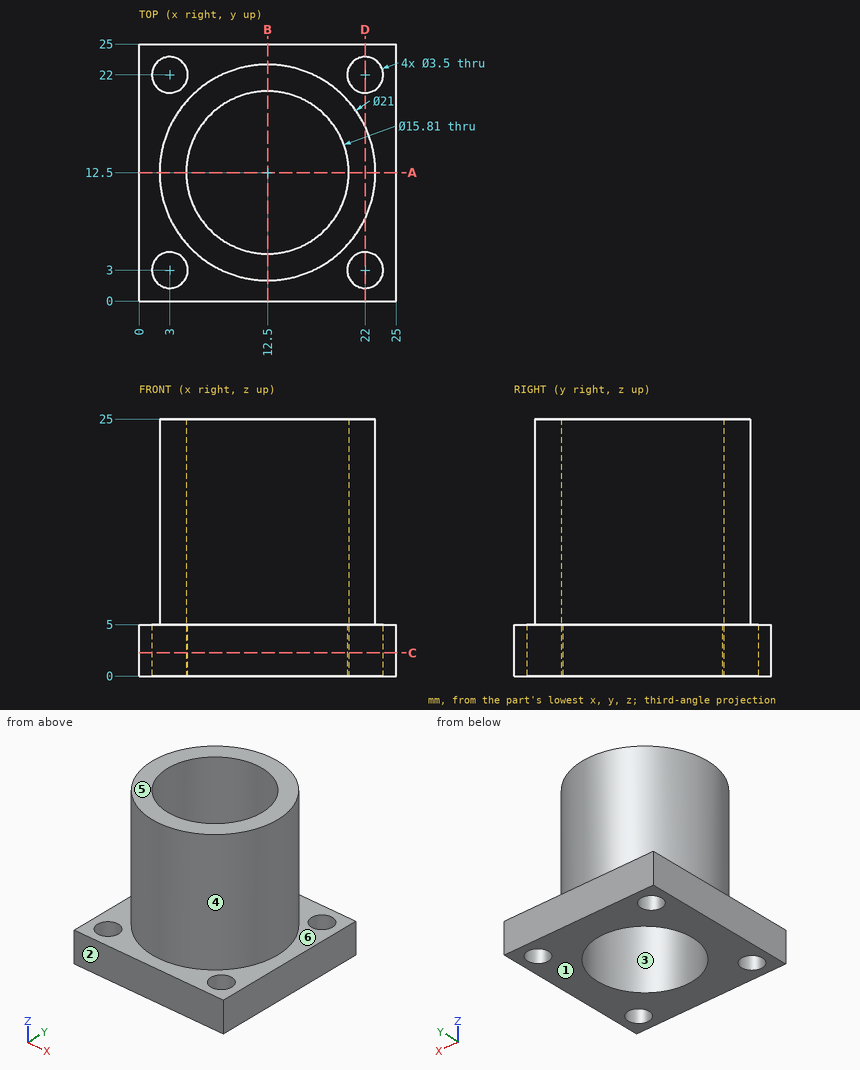
Verification items for this drawing (mm, ordinates from the low corner). A direction names the side the tool comes from. Give positions to 0.01 mm unless a question says otherwise; leave off trailing zeros. Order: outer loops, then holes, each group sorted by start corner. A loop starts at its lowest first (then second) coordinate and runs counter-clockwise, first axis right, second up. Notation, with made-up numbers: M 26,43.5 L 70,43.5 A21 ccw 70,47.5 Z; hole C -31,-24.5 d4. An arc over 180 degrees is marked long. Use a Markdown table: item, result.
Item 1: Tool access check on the marked faces 5 and 6. Record the directions out of +Z, -Z, +X, -X, +Y, -Y that give a thin tool (end or side, any length) a straight path to the whole face; none if there is none.
Answers follow:
| item | result |
|---|---|
| face 5 | +Z, +X, -X, +Y, -Y |
| face 6 | +Z |
Item 2: Section check D-D (x = 22). Record the cut outline in (y, z), and give its area (3 significant figures).
Answers follow:
| item | result |
|---|---|
| outline | M 0,0 L 1.25,0 L 1.25,5 L 0,5 Z; M 4.75,0 L 20.25,0 L 20.25,5 L 16.97,5 L 16.97,25 L 8.03,25 L 8.03,5 L 4.75,5 Z; M 23.75,0 L 25,0 L 25,5 L 23.75,5 Z |
| area | 269 mm2 |
Item 3: Section check C-C (z = 2.25). Record the cut outline in (x, y) (3 decimals).
Answers follow:
| item | result |
|---|---|
| outline | M 0,0 L 25,0 L 25,25 L 0,25 Z; hole C 3,3 d3.5; hole C 3,22 d3.5; hole C 12.5,12.5 d15.81; hole C 22,3 d3.5; hole C 22,22 d3.5 |
Item 4: Section check A-A (y = 12.5). Record the cut outline in (x, z) (3 decimals).
Answers follow:
| item | result |
|---|---|
| outline | M 0,0 L 4.595,0 L 4.595,25 L 2,25 L 2,5 L 0,5 Z; M 20.405,0 L 25,0 L 25,5 L 23,5 L 23,25 L 20.405,25 Z |
Item 5: Depth check by flat-ended pin: P1, Ø5, axis at y = 13, z = 17, coming from the +X side; P2, Ø1.5, axis at x = 22, y = 5.5, coming from the +Z side; P3, Ø2, axis at x = 11, z = 18, coming from the -Y side; P4, Ø12.5, axis at x = 12.5, y = 12.5, coming from the -Z side. Enter the tip coordinate at first touch or a pass-through.
Answers follow:
| item | result |
|---|---|
| P1 | stops at x = 23 |
| P2 | stops at z = 5 |
| P3 | stops at y = 2.01 |
| P4 | passes through |
Item 6: Material ranges on line 1 along Y through (x, z) = (3, 2); line 2 along Y through (x, z) = (1.5, 2.5); line 3 along Y through (x, z) = (12.5, 13) (3 decimals), recorded low to high.
Answers follow:
| item | result |
|---|---|
| line 1 | y = 0 to 1.25, 4.75 to 20.25, 23.75 to 25 |
| line 2 | y = 0 to 2.1, 3.9 to 21.1, 22.9 to 25 |
| line 3 | y = 2 to 4.595, 20.405 to 23 |
Item 7: Draft check along Y on the marked faces 1, 2, 3 and 4. Enter one of: +Y half, -Y half, draft (parallel to the pull), parting line (faces both ways), or undercut.
Answers follow:
| item | result |
|---|---|
| face 1 | draft |
| face 2 | -Y half |
| face 3 | undercut |
| face 4 | parting line |
